Check sheet for the modelled part. Datum: model origin and axes. Units: mm. A direction names the side the tool comes from. Round coordinates to 2 decimals unless told otherwise and drop trailing zeros. Write each loop counter-clockwise with the first axis right and the second up, starting at its lowest first coordinate (ties: lowest second). Pieces come first, ordered by that corner, then holes. Notation, with made-up numbers: (27.25, 43) - (51.25, 43) arc R25 ccw to (51.25, 68) - close; hole circle Ø4 at (40.25, 38.5). An arc over 180 degrees is marked (long way). Answer as a JSON object with one key per item and string values. Group by question number.
Item 1: Sectioned sample at A-A on y = 0. Record the boundary of the cut face in (x, z), plus the area to 3 significant figures.
Item 2: Thickness scan on line 1 (Y direction, x = -1, z = -8.5); line 2 (Y direction, x = -4.5, z = 8.5); line 3 (Z direction, x = -1.5, y = 0). Record the ranges inside material, lowest first.
Item 3: Set-up check for faces 4 (the flat face through (-1.651, 0, 0)), 5 (the cylindrical face through (-3.13, -0.39, -17.61)): record each of +Z, -Z, +X, -X, +Y, -Y from which the full face is reachable in a straight line by a thin tool's end or side.
Item 4: Sectioned sample at D-D on y = -16. Record the boundary of the cut face in (x, z), plus the area to 3 significant figures.
Item 5: Sectioned sample at C-C on x = -4.5. Count the separate pieces of the cut face and the enclosed holes in it, plus the area to 3 significant figures.
Item 6: Gauge pin test, flat ends, axial feed: P1, Ø2, axis at y = 13.75, z = -7.94, coming from the +X side; P2, Ø1, axis at x = -4, y = -12, coming from the +Z side; P3, Ø11, axis at y = -2.5, z = 2, coming from the +X side; P4, Ø2, axis at x = -3.5, z = -4.5, coming from the -Y side. Record the tip position at first contact, or that the pin passes through.
Item 7: Release check for a two-part mould opening along Z. For faces 1 (the cylindrical face through (-3.13, -0.39, 14.14)), 2 (the cylindrical face through (-3.22, 11.59, -15.12)), 3 (the flat face through (-6.35, 0, 0)) record: pulls with the +Z half, pulls with the -Z half, needs draft (parallel to the pull), parting line crosses it, or undercut.
Item 8: Sectioned sample at B-B on z = 0. Record the boundary of the cut face in (x, y), plus the area to 3 significant figures.
```python
from build123d import *

# Parameters (mm, degrees)
F2_R     = 1.778
F3_DEPTH = 6.351


with BuildPart() as f1:
    # F0 (on Front) → F1 (revolve)
    with BuildSketch(Plane.XZ):
        Polygon((-1.651, 11.049), (0, 12.7), (0, 19.05), (-6.35, 19.05), (-6.35, 0), (-1.651, 0), align=None)
    revolve(axis=Axis((-4.0005, 0, 0), (1, 0, 0)))

    # F2 (on Right) → F3 (cut, through all)
    with BuildSketch(Plane.YZ):
        with Locations((0, 15.875)):
            Circle(F2_R)
        with Locations((-13.748153, 7.9375)):
            Circle(F2_R)
        with Locations((-13.748153, -7.9375)):
            Circle(F2_R)
        with Locations((0, -15.875)):
            Circle(F2_R)
        with Locations((13.748153, -7.9375)):
            Circle(F2_R)
        with Locations((13.748153, 7.9375)):
            Circle(F2_R)
    extrude(amount=-F3_DEPTH, mode=Mode.SUBTRACT)


solid = f1.part
```
Completed:
{
 "1": {"outline": "(-6.35, -19.05) - (0, -19.05) - (0, -17.65) - (-6.35, -17.65) - close; (-6.35, -14.1) - (0, -14.1) - (0, -12.7) - (-1.65, -11.05) - (-1.65, 11.05) - (0, 12.7) - (0, 14.1) - (-6.35, 14.1) - close; (-6.35, 17.65) - (0, 17.65) - (0, 19.05) - (-6.35, 19.05) - close", "area": "158 mm²"},
 "2": {"line 1": "-17.05 to -15.43, -12.06 to -8.04, 8.04 to 12.06, 15.43 to 17.05", "line 2": "-17.05 to -15.43, -12.06 to 12.06, 15.43 to 17.05", "line 3": "-19.05 to -17.65, -14.1 to -11.2, 11.2 to 14.1, 17.65 to 19.05"},
 "3": {"face 4": "+X", "face 5": "+X, -X"},
 "4": {"outline": "(-6.35, -10.34) - (0, -10.34) - (0, 10.34) - (-6.35, 10.34) - close", "area": "131 mm²"},
 "5": {"separate pieces": "1", "enclosed holes": "6", "area": "1,080 mm²"},
 "6": {"P1": "through", "P2": "z = 15.19", "P3": "x = -1.65", "P4": "y = -18.73"},
 "7": {"face 1": "undercut", "face 2": "parting line crosses it", "face 3": "needs draft"},
 "8": {"outline": "(-6.35, -19.05) - (0, -19.05) - (0, -12.7) - (-1.65, -11.05) - (-1.65, 11.05) - (0, 12.7) - (0, 19.05) - (-6.35, 19.05) - close", "area": "203 mm²"}
}
